Read the model definition and answer for the solid it produces. Units are mm, in the model's axes. Face numbers are marked on the shaded views. A direction names the side the tool comes from. Give positions to 0.01 mm unless a question says otherwise; leave off trailing zeros. Order: outer loops, then holes, each group sorted by start corner. A loop starts at its lowest first (then second) coordinate and runs counter-clockwise, first axis right, second up. Notation, with made-up numbers: M 67,4.25 L 117,4.25 A27 ccw 117,29.25 Z; hole C -20,43.25 d4. An arc over 180 degrees is marked long. One line per item, written item: value.
Autodesk Inventor part; units mm, degrees
ref_plane "Work Plane1" through (0, 0, 0) normal (1, 0, 0) x (0, 1, 0)
ref_plane "XZ Plane" through (0, 0, 0) normal (0, 1, 0) x (-1, 0, 0)
ref_plane "XY Plane" through (0, 0, 0) normal (0, 0, 1) x (1, 0, 0)
ref_plane "Work Plane1" through (0, 0, 0) normal (1, 0, 0) x (0, 1, 0)
sketch "Sketch3" plane through (0, 0, 0) normal (1, 0, 0) x (0, 1, 0)
  line L0 (0, 0) -> (0, 14)
  line L1 (0, 14) -> (-5, 14)
  arc A0 (-9, 10) -> (-5, 14) centre (-9, 14) ccw
  line L2 (-9, 10) -> (-17.5, 10)
  line L3 (-17.5, 10) -> (-17.5, 7)
  line L4 (-17.5, 7) -> (-9, 7)
  line L5 (-9, 7) -> (-9, 0)
  line L6 (-9, 0) -> (0, 0)
  dimension "d10" = 4
  dimension "d11" = 3
  dimension "d12" = 35
  dimension "d13" = 7
  dimension "d14" = 18
revolve "Revolution2" add sketch "Sketch3" angle 360 about axis through (0, 0, 0) along (0, 0, 1)
sketch "Sketch4" plane through (0, 0, 14) normal (0, 0, 1) x (1, 0, 0)
  circle A0 centre (0, 0) radius 5
  point P0 (0, 0)
hole "Hole1" at (0, 0, 14) direction (0, 0, -1) diameter 6.647 depth 8
sketch "Sketch5" plane through (0, 0, 0) normal (0, 0, -1) x (-1, 0, 0)
  circle A0 centre (0, 0) radius 9
  point P0 (0, 0)
hole "Hole2" at (0, 0, 0) direction (0, 0, 1) diameter 5 depth 6
sketch "Sketch6" plane through (0, 0, 10) normal (0, 0, 1) x (1, 0, 0)
  line L0 (0, 0) -> (0, 20.3424) construction
  circle A0 centre (0, 0) radius 2.5
  line L1 (0, 0) -> (-11.8721, 20.5631) construction
  circle A1 centre (0, 0) radius 5
  circle A2 centre (0, 0) radius 14.5 construction
  point P0 (-7.25, 12.5574)
  dimension "d31" = 29
  dimension "d30" = 30
hole "Hole3" at (-7.25, 12.5574, 10) direction (0, 0, -1) diameter 3 depth 3
pattern_circular "Circular Pattern1" count 6 over 360 about axis through (0, 0, 8.5) along (0, 0, 1) of "Hole3"
properties part number "156" material "Gold"
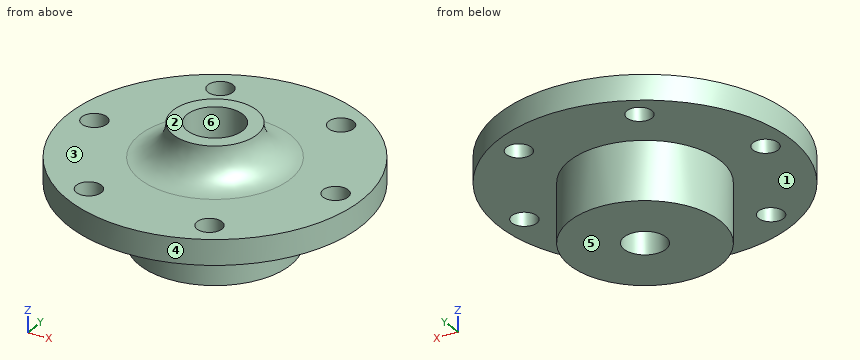
1) Find section C-C, the plane z = 9.25. Write down the section's boundary in (x, y).
Reported:
outline: C 0,0 d35; hole C -14.5,0 d3; hole C -7.25,-12.56 d3; hole C -7.25,12.56 d3; hole C 0,0 d6.65; hole C 7.25,-12.56 d3; hole C 7.25,12.56 d3; hole C 14.5,0 d3
2) Find section A-A, the plane y = 0. Write down the section's boundary in (x, z), plus the area to 3 significant figures.
Reported:
outline: M -17.5,7 L -16,7 L -16,10 L -17.5,10 Z; M -13,7 L -9,7 L -9,0 L -2.5,0 L -2.5,6 L -3.32,6 L -3.32,14 L -5,14 A4 cw -9,10 L -13,10 Z; M 2.5,0 L 9,0 L 9,7 L 13,7 L 13,10 L 9,10 A4 cw 5,14 L 3.32,14 L 3.32,6 L 2.5,6 Z; M 16,7 L 17.5,7 L 17.5,10 L 16,10 Z
area: 177 mm^2
3) Which of the six approach directions +Z, -Z, +X, -X, +Y, -Y give full straight-line access (tool end or side, diameter ignored) to the marked faces 1, 2 and 3?
Reported:
face 1: -Z
face 2: +Z, +X, -X, +Y, -Y
face 3: +Z
4) Find section B-B, the plane x = 0. Write down the section's boundary in (y, z), plus the area to 3 significant figures.
Reported:
outline: M -17.5,7 L -9,7 L -9,0 L -2.5,0 L -2.5,6 L -3.32,6 L -3.32,14 L -5,14 A4 cw -9,10 L -17.5,10 Z; M 2.5,0 L 9,0 L 9,7 L 17.5,7 L 17.5,10 L 9,10 A4 cw 5,14 L 3.32,14 L 3.32,6 L 2.5,6 Z
area: 195 mm^2
5) Determine the mould class of the marked faces 4, 5 and 6 for opening direction X: +X half, -X half, draft (parallel to the pull), parting line (faces both ways), or undercut.
Reported:
face 4: parting line
face 5: draft
face 6: undercut
6) Consider probe 1 along X at (y, z) = (0, 2.15); probe 2 along X at (y, z) = (12, 9.5); probe 3 along X at (y, z) = (0.5, 11.5). Determine where each line is inside the solid, lowest interval first.
Reported:
probe 1: x = -9 to -2.5, 2.5 to 9
probe 2: x = -12.74 to -8.64, -5.86 to 5.86, 8.64 to 12.74
probe 3: x = -5.86 to -3.29, 3.29 to 5.86
7) Find section D-D, the plane z = 1.5. Write down the section's boundary in (x, y).
Reported:
outline: C 0,0 d18; hole C 0,0 d5
8) Each of these flat-tipped pins is pushed along its axis until it touches: pin 1 Ø4 at (x, y) = (-9, 11.5) entering from -Z; pin 2 Ø5 at (y, z) = (5, 4) entering from +X; pin 3 Ø5.5 at (x, y) = (0, 0) entering from +Z. Where does it stop, or does it pass through?
Reported:
pin 1: stops at z = 7
pin 2: stops at x = 8.65
pin 3: stops at z = 6
